Model file for the job. Use its own axes, mm. A direction names the side the tool comes from. Round coordinates to 2 decimals unless told otherwise and drop trailing zeros. Loops run counter-clockwise (first coordinate to the right, second up) from the corner with the lowest first, then second, coordinate; pieces in that order, holes last. Notation, with made-up numbers: M -22.75,-24.5 L -4.75,-24.5 A15 ccw -4.75,-5.5 Z; hole C -11.5,-21 d5. An arc over 180 degrees is marked long. Answer in a Markdown table with one row per item.
from build123d import *

# Parameters (mm, degrees)
F0_W     = 150
F0_H     = 300
F1_DEPTH = 130
F2_T     = -10
F3_W     = 150
F3_H     = 10
F4_DEPTH = 100


with BuildPart() as f1:
    # F0 (on Top) → F1 (new body)
    with BuildSketch(Plane.XY):
        Rectangle(F0_W, F0_H)
    extrude(amount=F1_DEPTH)

    # F2
    f2_openings = [f1.faces().sort_by_distance(p)[0] for p in [
        (0, 0, 130),
    ]]
    offset(amount=F2_T, openings=f2_openings)

    # F3 (on face) → F4 (join)
    with BuildSketch(Plane.XY.offset(130)):
        with Locations((0, -145)):
            Rectangle(F3_W, F3_H)
    extrude(amount=F4_DEPTH)


solid = f1.part
1. Pin check, flat tips, straight feed: pin 1 (3 mm diameter, centred on x = -52.5, y = -87.5, fed in from +Z); pin 2 (1.5 mm diameter, centred on x = 45.5, z = 172.5, fed in from +Y). Stop position of each tip, or through.
Verdict:
| item | result |
|---|---|
| pin 1 | stops at z = 10 |
| pin 2 | stops at y = -140 |
2. Mould opens along X. For faces 4 (the flat face through (-65, -2, 69)), 5 (the flat face through (-1, 2, 0)), 6 (the flat face through (-75, -2, 62)) say: +X half, -X half, draft (parallel to the pull), parting line (faces both ways), or undercut.
Verdict:
| item | result |
|---|---|
| face 4 | undercut |
| face 5 | draft |
| face 6 | -X half |
3. Saw through at C-C (x = 50.5). Write the cut outline in (y, z).
Verdict:
| item | result |
|---|---|
| outline | M -150,0 L 150,0 L 150,130 L 140,130 L 140,10 L -140,10 L -140,230 L -150,230 Z |
4. Wall check: probe 1 along X at (y, z) = (-123, 82); probe 2 along Y at (x, z) = (-18, 38.5); probe 3 along Y at (x, z) = (20, 215.5). Give the ranges that are in metal, low to high.
Verdict:
| item | result |
|---|---|
| probe 1 | x = -75 to -65, 65 to 75 |
| probe 2 | y = -150 to -140, 140 to 150 |
| probe 3 | y = -150 to -140 |
5. Saw through at D-D (z = 151.5). Write the cut outline in (x, y), and give its area (3 significant figures).
Verdict:
| item | result |
|---|---|
| outline | M -75,-150 L 75,-150 L 75,-140 L -75,-140 Z |
| area | 1,500 mm² |
6. Tool access for faces 1 (the flat face through (-67, 27, 130)), 2 (the flat face through (-1, 2, 10)), 3 (the flat face through (75, -2, 62)): list every direction of +Z, -Z, +X, -X, +Y, -Y with a clear straight run to the whole face (end or side of a thin tool).
Verdict:
| item | result |
|---|---|
| face 1 | +Z, +X, -X, +Y |
| face 2 | +Z |
| face 3 | +Z, -Z, +X, +Y, -Y |
7. Saw through at A-A (z = 24). Write the cut outline in (x, y).
Verdict:
| item | result |
|---|---|
| outline | M -75,-150 L 75,-150 L 75,150 L -75,150 Z; hole M -65,-140 L 65,-140 L 65,140 L -65,140 Z |
8. Saw through at B-B (y = 30). Write the cut outline in (x, z), and give its area (3 significant figures).
Verdict:
| item | result |
|---|---|
| outline | M -75,0 L 75,0 L 75,130 L 65,130 L 65,10 L -65,10 L -65,130 L -75,130 Z |
| area | 3,900 mm² |
